```python
from build123d import *

# Parameters (mm, degrees)
BOSS_EXTRUDE1_DEPTH = 31.75
SKETCH2_W           = 12.7
SKETCH2_H           = 25.4
CUT_EXTRUDE1_DEPTH  = 63.5
SKETCH3_W           = 15.875
SKETCH3_H           = 25.4
CUT_EXTRUDE2_DEPTH  = 19.05
SKETCH4_W           = 22.225
SKETCH4_H           = 25.4
CUT_EXTRUDE3_DEPTH  = 39.1


with BuildPart() as part:
    # Sketch1 → Boss-Extrude1 (new body, symmetric)
    with BuildSketch(Plane(origin=(0, 0, 0), x_dir=(0, 0, -1), z_dir=(1, 0, 0))):
        Polygon((-52.000801282, -26.427804487), (36.899198718, -26.427804487), (36.899198718, -4.202804487), (-26.600801282, 11.672195513), (-52.000801282, 11.672195513), align=None)
    extrude(amount=BOSS_EXTRUDE1_DEPTH, both=True)

    # Sketch2 → Cut-Extrude1 (cut)
    with BuildSketch(Plane(origin=(0, 11.672195513, 0), x_dir=(1, 0, 0), z_dir=(0, 1, 0))):
        with Locations((0, -39.300801282)):
            Rectangle(SKETCH2_W, SKETCH2_H)
    extrude(amount=-CUT_EXTRUDE1_DEPTH, mode=Mode.SUBTRACT)

    # Sketch3 → Cut-Extrude2 (cut)
    with BuildSketch(Plane(origin=(0, 11.672195513, 0), x_dir=(1, 0, 0), z_dir=(0, 1, 0))):
        with Locations((23.8125, -39.300801282)):
            Rectangle(SKETCH3_W, SKETCH3_H)
        with Locations((-14.2875, -39.300801282)):
            Rectangle(SKETCH3_W, SKETCH3_H)
    extrude(amount=-CUT_EXTRUDE2_DEPTH, mode=Mode.SUBTRACT)

    # Sketch4 → Cut-Extrude3 (cut, through all)
    with BuildSketch(Plane.XZ.offset(26.427804487)):
        with Locations((0, -24.199198718)):
            Rectangle(SKETCH4_W, SKETCH4_H)
    extrude(amount=-CUT_EXTRUDE3_DEPTH, mode=Mode.SUBTRACT)


solid = part.part
```
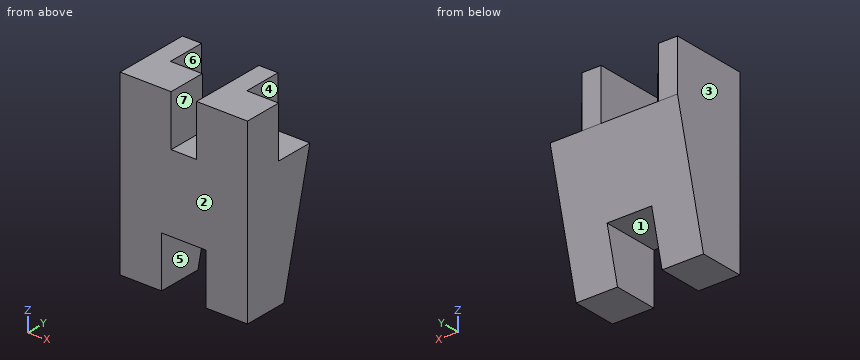
Design review of the part built by this model. Coordinates are the model's own, in mm. Face numbers are marked on the shaded views. A direction names the side the tool comes from. Coordinates: 2 decimals unless noted, no trailing zeros. Order: outer loops, then holes, each group sorted by start corner. A loop starts at its lowest first (then second) coordinate and runs counter-clockwise, first axis right, second up. Notation, with made-up numbers: M 89.5,-0.75 L 104.5,-0.75 A12 cw 104.5,22.25 Z; hole C 79.5,60.5 d8. An arc over 180 degrees is marked long. Answer as a JSON object with one key per item and string values. Group by question number.
1) Add section D-D, the plane z = -13. Write out the cut boundary in (x, y).
2) For pin 1 (8.5 mm diameter, centred on x = -14, y = 0.5, fed in from +Z); pin 2 (5.5 mm diameter, centred on y = 2.5, z = 44.5, fed in from +X) (3 decimals); pin 3 (1.5 mm diameter, centred on x = 11.5, z = 3.5, fed in from +Y), all flat-tipped, find the tip position at first contact; note any pin that passes through.
3) Add section C-C, the plane x = -8.5. Write out the cut boundary in (y, z), then the cut area to 3 significant figures.
4) Tool access review of the marked faces 4, 5, 6 and 7: name each direction out of +Z, -Z, +X, -X, +Y, -Y from which nothing blocks a thin tool from reaching the whole face with its end or side.
5) Add section B-B, the plane y = -19. Write out the cut boundary in (x, z), then the cut area to 3 significant figures.
6) Wall thickness on L1, parallel to X at y = -4, z = -25; L2, parallel to X at y = -10, z = 48; L3, parallel to Z at x = 8, y = -22.5: over which ranges is each line inside the solid? List them lowest first.
7) Add section A-A, the plane z = 34.5. Write out the cut boundary in (x, y) (3 decimals).
8) Mouldability with a two-part tool opening along X and no side actions: class the marked faces 1, 2 and 3 as pulls with the +X half, pulls with the -X half, needs draft (parallel to the pull), parting line crosses it, or undercut.
Computed values:
{
 "1": {"outline": "M -31.75,-26.43 L -11.11,-26.43 L -11.11,1.77 L -31.75,1.77 Z; M 11.11,-26.43 L 31.75,-26.43 L 31.75,1.77 L 11.11,1.77 Z"},
 "2": {"pin 1": "stops at z = 26.6", "pin 2": "stops at x = 15.875", "pin 3": "stops at y = 6.08"},
 "3": {"outline": "M -26.43,-11.5 L 2.15,-11.5 L 11.67,26.6 L -7.38,26.6 L -7.38,52 L -26.43,52 Z", "area": "1,750 mm^2"},
 "4": {"face 4": "+Z, +X, +Y", "face 5": "-Z, +Y, -Y", "face 6": "+Z, +Y", "face 7": "+Z, +Y, -Y"},
 "5": {"outline": "M -31.75,-36.9 L -11.11,-36.9 L -11.11,-11.5 L 11.11,-11.5 L 11.11,-36.9 L 31.75,-36.9 L 31.75,52 L 6.35,52 L 6.35,26.6 L -6.35,26.6 L -6.35,52 L -31.75,52 Z", "area": "4,760 mm^2"},
 "6": {"L1": "x = -31.75 to -11.11, 11.11 to 31.75", "L2": "x = -31.75 to -6.35, 6.35 to 31.75", "L3": "z = -11.5 to 52"},
 "7": {"outline": "M -31.75,-26.428 L -6.35,-26.428 L -6.35,-7.378 L -22.225,-7.378 L -22.225,11.672 L -31.75,11.672 Z; M 6.35,-26.428 L 31.75,-26.428 L 31.75,-7.378 L 15.875,-7.378 L 15.875,11.672 L 6.35,11.672 Z"},
 "8": {"face 1": "undercut", "face 2": "needs draft", "face 3": "pulls with the -X half"}
}
